```python
from build123d import *

# Parameters (mm, degrees)
RAIL_PROFILE_DEPTH             = 100
CBORE_FOR_M3_SHCS1_D           = 3.5
CBORE_FOR_M3_SHCS1_CBORE_D     = 6
CBORE_FOR_M3_SHCS1_CBORE_DEPTH = 4.5
FILL_START                     = -2.000000001
FILL_PATTERN1_OUTLINE_R        = 3
FILL_PATTERN1_DEPTH            = 4.5
FILL_START_2                   = -5.5
FILL_PATTERN1_2_OUTLINE_R      = 1.75
FILL_PATTERN1_2_DEPTH          = 3.499999999


# Read off the part's stored shape, not the designer's step: Fill Pattern1
with BuildPart() as part:
    # Sketch1 → RAIL PROFILE (new, symmetric)
    with BuildSketch(Plane.XY):
        with BuildLine():
            Line((-5.982334879, -1.370069213), (-5.982334879, -5.001472146))
            Line((-5.982334879, -5.001472146), (-5.483807025, -5.499999999))
            Line((-5.483807025, -5.499999999), (1.595289228, -5.499999999))
            ThreePointArc((1.595289228, -5.499999999), (1.994111552, -5.300588838), (2.392933875, -5.5))
            Line((2.392933875, -5.5), (5.483807024, -5.5))
            Line((5.483807024, -5.5), (5.982334878, -5.001472147))
            Line((5.982334878, -5.001472147), (5.982334878, -1.370069213))
            ThreePointArc((5.982334878, -1.370069213), (5.940056641, -1.231182813), (5.82756375, -1.139410101))
            ThreePointArc((5.82756375, -1.139410101), (5.497041405, -0.930122348), (5.251697363, -0.625405104))
            ThreePointArc((5.251697363, -0.625405104), (5.169975597, -0.541388466), (5.058890009, -0.504008866))
            Line((5.058890009, -0.504008866), (4.71429032, -0.473860299))
            ThreePointArc((4.71429032, -0.473860299), (4.552238438, -0.393945155), (4.486751147, -0.225544865))
            Line((4.486751147, -0.225544865), (4.486751147, 0.225544865))
            ThreePointArc((4.486751147, 0.225544865), (4.552238438, 0.393945155), (4.71429032, 0.473860299))
            Line((4.71429032, 0.473860299), (5.079776582, 0.505836204))
            ThreePointArc((5.079776582, 0.505836204), (5.187925163, 0.5413949), (5.268982803, 0.621333598))
            ThreePointArc((5.268982803, 0.621333598), (5.511607978, 0.899707672), (5.82756375, 1.09083865))
            ThreePointArc((5.82756375, 1.09083865), (5.940040963, 1.182638806), (5.982312115, 1.321532803))
            Line((5.982312115, 1.321532803), (5.982321902, 2.00145917))
            Line((5.982321902, 2.00145917), (5.483807025, 2.499999999))
            Line((5.483807025, 2.499999999), (-5.483807026, 2.499999999))
            Line((-5.483807026, 2.499999999), (-5.982321903, 2.00145917))
            Line((-5.982321903, 2.00145917), (-5.982321903, 1.32884687))
            ThreePointArc((-5.982321903, 1.32884687), (-5.942177076, 1.185718341), (-5.827697321, 1.090893402))
            ThreePointArc((-5.827697321, 1.090893402), (-5.511663234, 0.899754111), (-5.268982805, 0.621333597))
            ThreePointArc((-5.268982805, 0.621333597), (-5.187925164, 0.541394898), (-5.079776582, 0.505836204))
            Line((-5.079776582, 0.505836204), (-4.71429032, 0.473860299))
            ThreePointArc((-4.71429032, 0.473860299), (-4.552238438, 0.393945155), (-4.486751147, 0.225544865))
            Line((-4.486751147, 0.225544865), (-4.486751147, -0.225544865))
            ThreePointArc((-4.486751147, -0.225544865), (-4.552238438, -0.393945155), (-4.71429032, -0.473860299))
            Line((-4.71429032, -0.473860299), (-5.058890009, -0.504008866))
            ThreePointArc((-5.058890009, -0.504008866), (-5.169975597, -0.541388466), (-5.251697363, -0.625405104))
            ThreePointArc((-5.251697363, -0.625405104), (-5.499180752, -0.921502608), (-5.828043428, -1.123421157))
            ThreePointArc((-5.828043428, -1.123421157), (-5.944906256, -1.221900029), (-5.982334879, -1.370069213))
        make_face()
    extrude(amount=RAIL_PROFILE_DEPTH, both=True)

    # CBORE for M3 SHCS1 (through all)
    with Locations(Plane(origin=(0, 2.499999999, 0), x_dir=(1, 0, 0), z_dir=(0, 1, 0))):
        with Locations((0, 90)):
            cbore_for_m3_shcs1 = CounterBoreHole(CBORE_FOR_M3_SHCS1_D / 2, CBORE_FOR_M3_SHCS1_CBORE_D / 2, CBORE_FOR_M3_SHCS1_CBORE_DEPTH)

    # M3 END MIRROR: CBORE for M3 SHCS1 across plane
    add(cbore_for_m3_shcs1.mirror(Plane.XY), mode=Mode.SUBTRACT)

    # Fill Pattern1 outline → Fill Pattern1 (cut)
    with BuildSketch(Plane(origin=(0, 0, 0), x_dir=(1, 0, 0), z_dir=(0, 1, 0)).offset(FILL_START)):
        with Locations((0, 65)):
            Circle(FILL_PATTERN1_OUTLINE_R)
        with Locations((0, 40)):
            Circle(FILL_PATTERN1_OUTLINE_R)
        with Locations((0, 15)):
            Circle(FILL_PATTERN1_OUTLINE_R)
        with Locations((0, -10)):
            Circle(FILL_PATTERN1_OUTLINE_R)
        with Locations((0, -35)):
            Circle(FILL_PATTERN1_OUTLINE_R)
        with Locations((0, -60)):
            Circle(FILL_PATTERN1_OUTLINE_R)
    extrude(amount=FILL_PATTERN1_DEPTH, mode=Mode.SUBTRACT)

    # Fill Pattern1 2 outline → Fill Pattern1 2 (cut)
    with BuildSketch(Plane(origin=(0, 0, 0), x_dir=(1, 0, 0), z_dir=(0, 1, 0)).offset(FILL_START_2)):
        with Locations((0, 65)):
            Circle(FILL_PATTERN1_2_OUTLINE_R)
        with Locations((0, 40)):
            Circle(FILL_PATTERN1_2_OUTLINE_R)
        with Locations((0, 15)):
            Circle(FILL_PATTERN1_2_OUTLINE_R)
        with Locations((0, -10)):
            Circle(FILL_PATTERN1_2_OUTLINE_R)
        with Locations((0, -35)):
            Circle(FILL_PATTERN1_2_OUTLINE_R)
        with Locations((0, -60)):
            Circle(FILL_PATTERN1_2_OUTLINE_R)
    extrude(amount=FILL_PATTERN1_2_DEPTH, mode=Mode.SUBTRACT)


solid = part.part
```
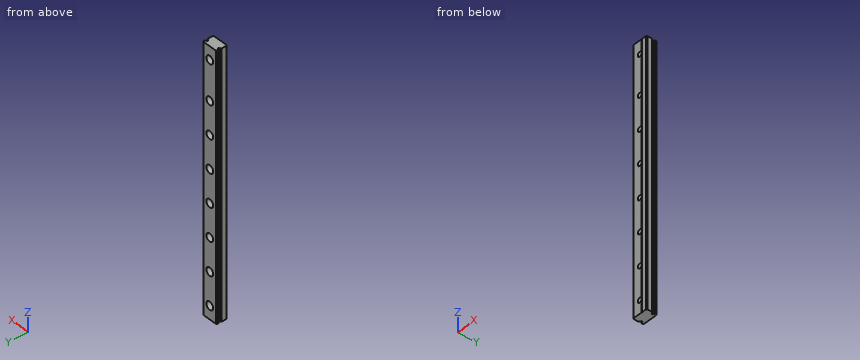
Geometry: final body of the model. Coordinates: model frame, mm. Coordinates: 2 decimals unless noted, no trailing zeros. Put each result on its own line as item: value.
(1) Material intervals for probe 1 along X at (y, z) = (1.35, 35); probe 2 along Y at (x, z) = (-5.25, 58); probe 3 along X at (y, z) = (-4.05, -40), sorted ascending.
Answer sheet:
probe 1: x = -5.98 to -3, 3 to 5.98
probe 2: y = -5.5 to -0.62, 0.6 to 2.5
probe 3: x = -5.98 to -1.75, 1.75 to 5.98
(2) Cut plane A-A on y = -3.75. State how many separate pieces and enclosed holes the cut face has, then the cut area to 3 significant figures.
Answer sheet:
separate pieces: 1
enclosed holes: 8
area: 2,320 mm^2
(3) First-contact query: pin 1 (1.8 mm diameter, centred on x = 0.5, z = 35, fed in from +Y); pin 2 (6.5 mm diameter, centred on x = -0.5, z = -39.5, fed in from +Y); pin 3 (1.8 mm diameter, centred on x = 1.5, z = -89.5, fed in from +Y). Flat tips, straight axial feed; report the tip coordinate or a pass-through.
Answer sheet:
pin 1: passes through
pin 2: stops at y = 2.5
pin 3: stops at y = -2
